Can you work these out from the model? Positions are in its coordinate system, mm. Give positions to 0.01 mm unless a question says otherwise; leave off trailing zeros. Order: outer loops, then holes, each group sorted by start corner. A loop starts at its lowest first (then second) coordinate and runs counter-clockwise, first axis right, second up. Notation, with made-up numbers: (47, -28.75) - (88, -28.75) arc R17 cw to (88, -4.75) - close; hole circle Ø11 at (36, 25.25). An arc over 180 degrees is marked (long way). Write each question's results on one line, items separated by ' | '. Start each with the question number.
from build123d import *

# Parameters (mm, degrees)
BOSS_EXTRUDE1_DEPTH = 2.032


with BuildPart() as part:
    # Sketch1 → Boss-Extrude1 (new body)
    with BuildSketch(Plane.XY):
        Polygon((221.544444444, 0), (218.722222222, -50.8), (2.822222222, -50.8), (0, 0), align=None)
        Polygon((212.372222222, -50.8), (9.172222222, -50.8), (25.047222222, -520.7), (196.497222222, -520.7), align=None)
    extrude(amount=BOSS_EXTRUDE1_DEPTH)


solid = part.part
Q1. If we section it at C-C (y = -430): Please give me the cut outline in (x, z), plus the area to 3 significant figures.
Q2. If we section it at A-A (z = 1.4): Please give me the cut outline in (x, y), plus the area to 3 significant figures.
Q3. Will these pins go through, and if not, where does the flat tip stop? P1, Ø1, axis at y = -62.5, z = 2, coming from the +X side; P2, Ø1, axis at x = 5.5, z = 1, coming from the -Y side.
Q4. If I drill on probe 1 along X at (y, z) = (-49.5, 1.1); probe 2 along X at (y, z) = (-279, 0.3), over which ranges is the centre line in solid material (lowest first)? Write a range as from..to.
Q5. If we section it at B-B (y = -150.5): Please give me the cut outline in (x, z).
Findings below:
1) outline: (21.98, 0) - (199.56, 0) - (199.56, 2.03) - (21.98, 2.03) - close | area: 361 mm2
2) outline: (0, 0) - (2.82, -50.8) - (9.17, -50.8) - (25.05, -520.7) - (196.5, -520.7) - (212.37, -50.8) - (218.72, -50.8) - (221.54, 0) - close | area: 99,100 mm2
3) P1: stops at x = 211.99 | P2: stops at y = -50.8
4) probe 1: x = 2.75..218.79 | probe 2: x = 16.88..204.66
5) outline: (12.54, 0) - (209, 0) - (209, 2.03) - (12.54, 2.03) - close
